from build123d import *

# Parameters (mm, degrees)
F0_W      = 50
F0_H      = 35
F1_DEPTH  = 6
F2_W      = 14
F2_H      = 35
F3_DEPTH  = 15
F4_W      = 15
F4_H      = 13.216582
F5_DEPTH  = 25
F6_R      = 4.5
F7_DEPTH  = 41.5
F8_W      = 6
F8_H      = 35
F9_DEPTH  = 9.7
F11_DEPTH = 36.8


with BuildPart() as f1:
    # F0 (on Top) → F1 (new body)
    with BuildSketch(Plane.XY):
        Rectangle(F0_W, F0_H)
    extrude(amount=F1_DEPTH)

    # F2 (on face) → F3 (join)
    with BuildSketch(Plane.XY.offset(6)):
        with Locations((-18, 0)):
            Rectangle(F2_W, F2_H)
    extrude(amount=F3_DEPTH)

    # F4 (on face) → F5 (cut)
    with BuildSketch(Plane.YZ.offset(-11)):
        with Locations((0, 14.391709)):
            Rectangle(F4_W, F4_H)
    extrude(amount=-F5_DEPTH, mode=Mode.SUBTRACT)

    # F6 (on face) → F7 (cut)
    with BuildSketch(Plane.XZ.offset(17.5)):
        with Locations((-17.95, 14.500192)):
            Circle(F6_R)
    extrude(amount=-F7_DEPTH, mode=Mode.SUBTRACT)

    # F8 (on face) → F9 (join)
    with BuildSketch(Plane.XY.offset(6)):
        with Locations((22, 0)):
            Rectangle(F8_W, F8_H)
    extrude(amount=F9_DEPTH)

    # F10 (on face) → F11 (cut)
    with BuildSketch(Plane(origin=(0, 17.5, 0), x_dir=(-1, 0, 0), z_dir=(0, 1, 0))):
        Polygon((-22.35515, 10.7), (-25, 10.7), (-25, 7.547991), align=None)
    extrude(amount=-F11_DEPTH, mode=Mode.SUBTRACT)


solid = f1.part
Can you work these out from the model? Positions are in its coordinate system, mm. A direction names the side the tool comes from. Coordinates: 2 decimals unless noted, no trailing zeros. Loops run counter-clockwise (first coordinate to the right, second up) from the corner with the lowest first, then second, coordinate; pieces in that order, holes last. Notation, with made-up numbers: (65, 7.5) - (104, 7.5) arc R24 ccw to (104, 42.5) - close; hole circle Ø3 at (-40, -9). An arc over 180 degrees is marked (long way). Answer as a JSON object with one key per item and string values. Group by question number.
Item 1: If we section it at B-B (y = 3): List the corners of the cut face in (x, z) for me.
Item 2: If we section it at C-C (z = 13.5): List the corners of the cut face in (x, y) for me.
Item 3: For pin 1 (3 mm diameter, centred on x = 17, y = -8.5, fed in from +Z); pin 2 (5 mm diameter, centred on x = 20.5, y = -7.5, fed in from +Z); pin 3 (6 mm diameter, centred on x = -6.5, z = 16.5, fed in from -Y), each with a flat end and sliding along its axis, tell me the tip position at first contact or that it passes through.
Item 4: On a 3-axis mill with a long thin cutter (end or side, diameter ignored), from which of +Z, -Z, +X, -X, +Y, -Y can I reach the whole of each face in a straight line? I mean faces 1 (the face through (23.7, 0.2, 9.1)), 2 (the face through (4, 0, 6)), 3 (the face through (-18, 13, 21)), 4 (the face through (-22.446, 12.43, 14.698)), 5 (the face through (-18, 0, 7.783)). Say none if no direction works.
Item 5: If we section it at D-D (y = 15): List the corners of the cut face in (x, z) for me, plus the area to 3 significant figures.
Item 6: If we mould it in two halves opening along X, with no side actions, what happens to faces 6 (the face through (22, 0, 15.7)), 7 (the face through (-25, 0, 6)), 8 (the face through (-22.446, -12.57, 14.698))? For each: released by +X, released by -X, zero draft, split by the parting line, or undercut.
Item 7: If I drill on L1, parallel to X at y = 13.5, z = 14.25; L2, parallel to Z at x = -17.95, y = -14; L3, parallel to X at y = -2.5, z = 14.25, over which ranges is the centre line in solid material (lowest first)? Write a range as from..to.
Item 8: If we section it at A-A (x = -17.95): List the corners of the cut face in (y, z) for me, plus the area to 3 significant figures.
Returned:
{
 "1": {"outline": "(-25, 0) - (25, 0) - (25, 7.55) - (22.36, 10.7) - (25, 10.7) - (25, 15.7) - (19, 15.7) - (19, 6) - (-11, 6) - (-11, 7.78) - (-25, 7.78) - close"},
 "2": {"outline": "(-25, -17.5) - (-22.34, -17.5) - (-22.34, -7.5) - (-25, -7.5) - close; (-25, 7.5) - (-22.34, 7.5) - (-22.34, 17.5) - (-25, 17.5) - close; (-13.56, -17.5) - (-11, -17.5) - (-11, -7.5) - (-13.56, -7.5) - close; (-13.56, 7.5) - (-11, 7.5) - (-11, 17.5) - (-13.56, 17.5) - close; (19, -17.5) - (25, -17.5) - (25, 17.5) - (19, 17.5) - close"},
 "3": {"pin 1": "stops at z = 6", "pin 2": "stops at z = 15.7", "pin 3": "passes through"},
 "4": {"face 1": "+X, +Y, -Y", "face 2": "+Z, +Y, -Y", "face 3": "+Z, +X, -X, +Y, -Y", "face 4": "+Y, -Y", "face 5": "+Z, -X"},
 "5": {"outline": "(-25, 0) - (25, 0) - (25, 7.55) - (22.36, 10.7) - (25, 10.7) - (25, 15.7) - (19, 15.7) - (19, 6) - (-11, 6) - (-11, 21) - (-25, 21) - close; hole circle Ø9 at (-17.95, 14.5)", "area": "500 mm²"},
 "6": {"face 6": "zero draft", "face 7": "released by -X", "face 8": "undercut"},
 "7": {"L1": "x = -25..-22.44, -13.46..-11, 19..25", "L2": "z = 0..10, 19..21", "L3": "x = 19..25"},
 "8": {"outline": "(-17.5, 0) - (17.5, 0) - (17.5, 10) - (7.5, 10) - (7.5, 7.78) - (-7.5, 7.78) - (-7.5, 10) - (-17.5, 10) - close; (-17.5, 19) - (-7.5, 19) - (-7.5, 21) - (-17.5, 21) - close; (7.5, 19) - (17.5, 19) - (17.5, 21) - (7.5, 21) - close", "area": "357 mm²"}
}
